Check sheet for the modelled part. Datum: model origin and axes. Units: mm. Face numbers are marked on the shaded views. A direction names the side the tool comes from. Round coordinates to 2 decimals unless told otherwise and drop trailing zeros. Write each loop counter-clockwise with the first axis right and the second up, starting at its lowest first coordinate (ties: lowest second). Pieces come first, ordered by that corner, then holes.
Item 1: Cross-section at C-C on x = 0. Enter the section's corners in (y, z), plus the area to 3 significant figures.
Item 2: Tool access check on the marked faces 1 and 2. Record the directions out of +Z, -Z, +X, -X, +Y, -Y that give a thin tool (end or side, any length) a straight path to the whole face; none if there is none.
Item 3: Go/stop test with flat-tipped pins: pin 1 Ø3 at (x, y) = (24, 6.5) entering from -Z; pin 2 Ø1 at (x, z) = (-2.5, 5.5) entering from +Y. Record where each tip stops, or that it passes through.
Item 4: Cross-section at B-B on y = 7. Enter the section's corners in (x, z).
Item 5: Cross-section at D-D on x = 28. Enter the section's corners in (y, z), plus the area to 3 significant figures.
Item 6: Cross-section at A-A on x = 9. Enter the section's corners in (y, z).
Item 7: Material ranges on line 1 (X direction, y = 0.9, z = -18); line 2 (Z direction, x = 23, y = 2.5); line 3 (Z direction, x = -20, y = 3.75), recorded low to high.
Item 8: Release check for a two-part mould opening along Z. For the marked faces 3 and 4 record: +Z half, -Z half, draft (parallel to the pull), parting line (faces both ways), or undercut.
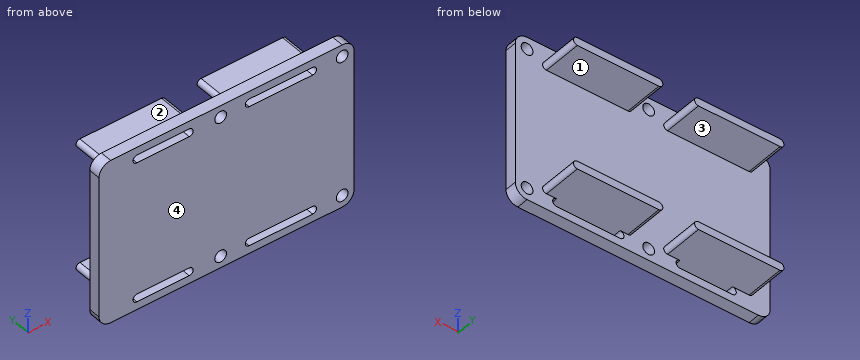
from build123d import *

# Parameters (mm, degrees)
SKETCH1_R           = 1.5
BOSS_EXTRUDE1_DEPTH = 3
BOSS_EXTRUDE2_DEPTH = 10


with BuildPart() as part:
    # Sketch1 → Boss-Extrude1 (new body)
    with BuildSketch(Plane(origin=(0, 0, 0), x_dir=(1, 0, 0), z_dir=(0, 1, 0))):
        with BuildLine():
            Line((0, -21), (31, -21))
            ThreePointArc((31, -21), (33.121320344, -20.121320344), (34, -18))
            Line((34, -18), (34, 18))
            ThreePointArc((34, 18), (33.121320344, 20.121320344), (31, 21))
            Line((31, 21), (0, 21))
            Line((0, 21), (-28, 21))
            ThreePointArc((-28, 21), (-30.121320344, 20.121320344), (-31, 18))
            Line((-31, 18), (-31, -18))
            ThreePointArc((-31, -18), (-30.121320344, -20.121320344), (-28, -21))
            Line((-28, -21), (0, -21))
        make_face()
        with Locations(Location((0, 18, 0), (0, 0, 270))):
            Circle(SKETCH1_R, mode=Mode.SUBTRACT)
        with Locations(Location((31, 18, 0), (0, 0, 270))):
            Circle(SKETCH1_R, mode=Mode.SUBTRACT)
        with Locations(Location((31, -18, 0), (0, 0, 270))):
            Circle(SKETCH1_R, mode=Mode.SUBTRACT)
        with Locations(Location((0, -18, 0), (0, 0, 270))):
            Circle(SKETCH1_R, mode=Mode.SUBTRACT)
        with BuildLine():
            Line((-21.341863145, 17), (-7.990756516, 17))
            ThreePointArc((-7.990756516, 17), (-6.990756516, 18), (-7.990756516, 19))
            Line((-7.990756516, 19), (-21.341863145, 19))
            ThreePointArc((-21.341863145, 19), (-22.341863145, 18), (-21.341863145, 17))
        make_face(mode=Mode.SUBTRACT)
        with BuildLine():
            Line((7.282100309, 17), (23.465259859, 17))
            ThreePointArc((23.465259859, 17), (24.465259859, 18), (23.465259859, 19))
            Line((23.465259859, 19), (7.282100309, 19))
            ThreePointArc((7.282100309, 19), (6.282100309, 18), (7.282100309, 17))
        make_face(mode=Mode.SUBTRACT)
        with BuildLine():
            Line((-21.341863145, -19), (-7.990756516, -19))
            ThreePointArc((-7.990756516, -19), (-6.990756516, -18), (-7.990756516, -17))
            Line((-7.990756516, -17), (-21.341863145, -17))
            ThreePointArc((-21.341863145, -17), (-22.341863145, -18), (-21.341863145, -19))
        make_face(mode=Mode.SUBTRACT)
        with BuildLine():
            Line((7.282100309, -19), (23.465259859, -19))
            ThreePointArc((23.465259859, -19), (24.465259859, -18), (23.465259859, -17))
            Line((23.465259859, -17), (7.282100309, -17))
            ThreePointArc((7.282100309, -17), (6.282100309, -18), (7.282100309, -19))
        make_face(mode=Mode.SUBTRACT)
    extrude(amount=BOSS_EXTRUDE1_DEPTH)

    # Sketch2 → Boss-Extrude2 (add)
    with BuildSketch(Plane(origin=(0, 3, 0), x_dir=(1, 0, 0), z_dir=(0, 1, 0))):
        with BuildLine():
            Line((-4.836170767, -15), (-25.624305917, -15))
            ThreePointArc((-25.624305917, -15), (-26.624305917, -16), (-25.624305917, -17))
            Line((-25.624305917, -17), (-4.836170767, -17))
            ThreePointArc((-4.836170767, -17), (-3.836170767, -16), (-4.836170767, -15))
        make_face()
        with BuildLine():
            ThreePointArc((-25.624305917, 17), (-26.624305917, 16), (-25.624305917, 15))
            Line((-25.624305917, 15), (-4.836170767, 15))
            ThreePointArc((-4.836170767, 15), (-3.836170767, 16), (-4.836170767, 17))
            Line((-4.836170767, 17), (-25.624305917, 17))
        make_face()
        with BuildLine():
            Line((26.046785566, -15), (5.262345151, -15))
            ThreePointArc((5.262345151, -15), (4.262345151, -16), (5.262345151, -17))
            Line((5.262345151, -17), (26.046785566, -17))
            ThreePointArc((26.046785566, -17), (27.046785566, -16), (26.046785566, -15))
        make_face()
        with BuildLine():
            ThreePointArc((5.262345151, 17), (4.262345151, 16), (5.262345151, 15))
            Line((5.262345151, 15), (26.046785566, 15))
            ThreePointArc((26.046785566, 15), (27.046785566, 16), (26.046785566, 17))
            Line((26.046785566, 17), (5.262345151, 17))
        make_face()
    extrude(amount=BOSS_EXTRUDE2_DEPTH)


solid = part.part
Response values:
1. outline: (0, -21) - (3, -21) - (3, -19.5) - (0, -19.5) - close; (0, -16.5) - (3, -16.5) - (3, 16.5) - (0, 16.5) - close; (0, 19.5) - (3, 19.5) - (3, 21) - (0, 21) - close
1. area: 108 mm2
2. face 1: +X, -X, +Y
2. face 2: +Y
3. pin 1: stops at z = -17
3. pin 2: stops at y = 3
4. outline: (-25.62, -17) - (-4.84, -17) arc R1 ccw to (-4.84, -15) - (-25.62, -15) arc R1 ccw to start; (-25.62, 15) - (-4.84, 15) arc R1 ccw to (-4.84, 17) - (-25.62, 17) arc R1 ccw to start; (5.26, -17) - (26.05, -17) arc R1 ccw to (26.05, -15) - (5.26, -15) arc R1 ccw to start; (5.26, 15) - (26.05, 15) arc R1 ccw to (26.05, 17) - (5.26, 17) arc R1 ccw to start
5. outline: (0, -21) - (3, -21) - (3, 21) - (0, 21) - close
5. area: 126 mm2
6. outline: (0, -21) - (3, -21) - (3, -19) - (0, -19) - close; (0, -17) - (13, -17) - (13, -15) - (3, -15) - (3, 15) - (13, 15) - (13, 17) - (0, 17) - close; (0, 19) - (3, 19) - (3, 21) - (0, 21) - close
7. line 1: x = -31 to -22.34, -6.99 to -1.5, 1.5 to 6.28, 24.47 to 29.5, 32.5 to 34
7. line 2: z = -21 to -19, -17 to 17, 19 to 21
7. line 3: z = -17 to -15, 15 to 17
8. face 3: undercut
8. face 4: draft
